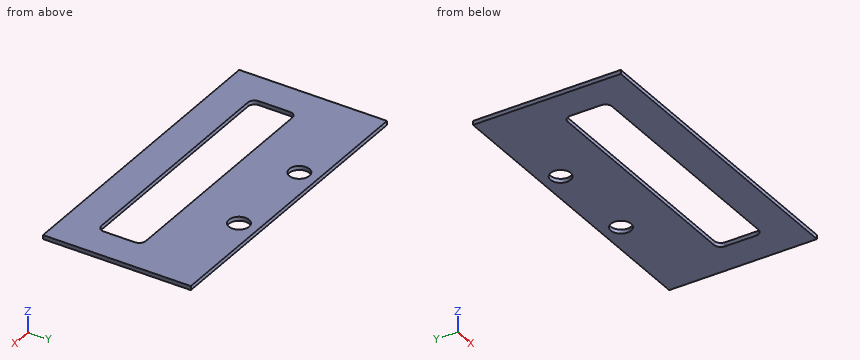
```python
from build123d import *

# Parameters (mm, degrees)
F0_W     = 228
F0_H     = 110
F1_DEPTH = 3
F2_W     = 180
F2_H     = 33
F3_DEPTH = 25
F4_R     = 5
F5_R     = 7.5
F6_DEPTH = 25


with BuildPart() as f1:
    # F0 (on Top) → F1 (new body)
    with BuildSketch(Plane.XY):
        with Locations((-114, 55)):
            Rectangle(F0_W, F0_H)
    extrude(amount=F1_DEPTH)

    # F2 (on face) → F3 (cut)
    with BuildSketch(Plane.XY.offset(3)):
        with Locations((-114, 41.5)):
            Rectangle(F2_W, F2_H)
    extrude(amount=-F3_DEPTH, mode=Mode.SUBTRACT)

    # F4
    f4_edges = [f1.edges().sort_by_distance(p)[0] for p in [
        (-24, 25, 1.5),
        (-24, 58, 1.5),
        (-204, 58, 1.5),
        (-204, 25, 1.5),
    ]]
    fillet(f4_edges, radius=F4_R)

    # F5 (on face) → F6 (cut)
    with BuildSketch(Plane(origin=(0, 0, 0), x_dir=(1, 0, 0), z_dir=(0, 0, -1))):
        with Locations((-148, -96)):
            Circle(F5_R)
        with Locations((-77.9, -96)):
            Circle(F5_R)
    extrude(amount=-F6_DEPTH, mode=Mode.SUBTRACT)


solid = f1.part
```
The listing builds one solid part. Answer for the finished solid, in the listing's coordinates (mm). Coordinates: 2 decimals unless noted, no trailing zeros. Loops run counter-clockwise (first coordinate to the right, second up) from the corner with the lowest first, then second, coordinate; pieces in that order, holes last. Notation, with made-up numbers: M 15.25,32 L 21.25,32 A22 cw 21.25,43 Z; hole C 8.25,-9.75 d2. An arc over 180 degrees is marked long. Answer as a JSON object with one key per item and string values. Group by question number.
Item 1: Section D-D (z = 1) is taken. Write down the section's boundary in (x, y), and give its area (3 significant figures).
Item 2: Section A-A (x = -148) is taken. Write down the section's boundary in (y, z).
Item 3: Consider L1, parallel to X at y = 96, z = 1.75; L2, parallel to Y at x = -77.9, z = 2.3; L3, parallel to Y at x = -57, z = 0.7. Determine where each line is inside the solid, lowest interval first.
Item 4: Section C-C (y = 96) is taken. Write down the section's boundary in (x, z).
Item 5: Section B-B (x = -182) is taken. Write down the section's boundary in (y, z), and give its area (3 significant figures).
Solved:
{
 "1": {"outline": "M -228,0 L 0,0 L 0,110 L -228,110 Z; hole M -204,30 A5 ccw -199,25 L -29,25 A5 ccw -24,30 L -24,53 A5 ccw -29,58 L -199,58 A5 ccw -204,53 Z; hole C -148,96 d15; hole C -77.9,96 d15", "area": "18,800 mm2"},
 "2": {"outline": "M 0,0 L 25,0 L 25,3 L 0,3 Z; M 58,0 L 88.5,0 L 88.5,3 L 58,3 Z; M 103.5,0 L 110,0 L 110,3 L 103.5,3 Z"},
 "3": {"L1": "x = -228 to -155.5, -140.5 to -85.4, -70.4 to 0", "L2": "y = 0 to 25, 58 to 88.5, 103.5 to 110", "L3": "y = 0 to 25, 58 to 110"},
 "4": {"outline": "M -228,0 L -155.5,0 L -155.5,3 L -228,3 Z; M -140.5,0 L -85.4,0 L -85.4,3 L -140.5,3 Z; M -70.4,0 L 0,0 L 0,3 L -70.4,3 Z"},
 "5": {"outline": "M 0,0 L 25,0 L 25,3 L 0,3 Z; M 58,0 L 110,0 L 110,3 L 58,3 Z", "area": "231 mm2"}
}
